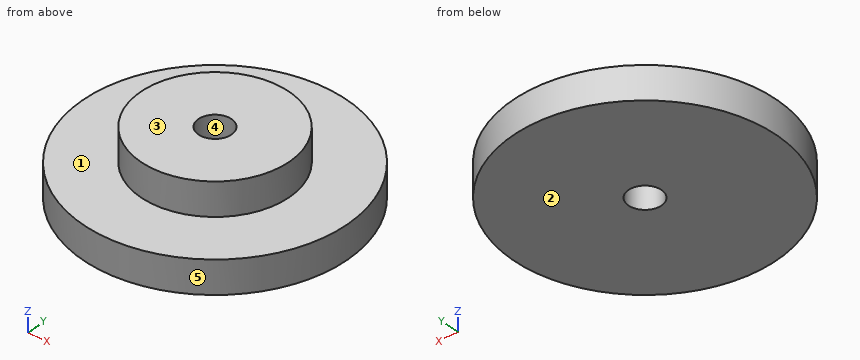
from build123d import *

# Parameters (mm, degrees)
F0_R     = 12.7
F0_R_2   = 7.14375
F1_DEPTH = 3.175
F0_R_3   = 1.5875
F2_DEPTH = 6.35
F3_DEPTH = 6.35


with BuildPart() as f1:
    # F0 (on Top) → F1 (new body)
    with BuildSketch(Plane.XY):
        Circle(F0_R)
        Circle(F0_R_2, mode=Mode.SUBTRACT)
    extrude(amount=F1_DEPTH)

    # F0 (on Top) → F2 (join)
    with BuildSketch(Plane.XY):
        Circle(F0_R_2)
        Circle(F0_R_3, mode=Mode.SUBTRACT)
    extrude(amount=F2_DEPTH)

    # F0 (on Top) → F3 (cut)
    with BuildSketch(Plane.XY):
        Circle(F0_R_3)
    extrude(amount=-F3_DEPTH, mode=Mode.SUBTRACT)


solid = f1.part
Build history of the part. All positions in model axes, mm. Face numbers are marked on the shaded views. A direction names the side the tool comes from. Coordinates: 2 decimals unless noted, no trailing zeros. Write each loop counter-clockwise with the first axis right and the second up, starting at its lowest first coordinate (ties: lowest second). Pieces come first, ordered by that corner, then holes.
(1) Cut at C-C on z = 1.75. List the corners of the cut face in (x, y) (1 decimal).
(2) 3-axis set-ups, long thin cutter, end or side, ignore diameter. For the marked faces 1 and 2: which of +Z, -Z, +X, -X, +Y, -Y reach the whole face in a straight line?
(3) Mould opens along X. For the marked faces 3, 4 and 5 say: pulls with the +X half, pulls with the -X half, needs draft (parallel to the pull), parting line crosses it, or undercut.
(4) Pin check, flat tips, straight feed: pin 1 Ø3 at (x, z) = (-7, 0.5) entering from -Y; pin 2 Ø1 at (x, y) = (0.5, 9) entering from +Z (3 decimals); pin 3 Ø1 at (y, z) = (9.5, 2.5) entering from +X. Stop position of each tip, or through.
(5) Drill centre lines: line 1 (Y direction, x = 0, z = 2.75); line 2 (Z direction, x = -6.75, y = -8.5) (3 decimals); line 3 (X direction, y = -10.5, z = 3). Where is each one in solid material? Low to high.
(6) Cut at D-D on x = 5.5. List the corners of the cut face in (y, z) (3 decimals).
Working result:
1. outline: circle Ø25.4 at (0, 0); hole circle Ø3.2 at (0, 0)
2. face 1: +Z
2. face 2: -Z, +X, -X, +Y, -Y
3. face 3: needs draft
3. face 4: undercut
3. face 5: parting line crosses it
4. pin 1: stops at y = -11.45
4. pin 2: stops at z = 3.175
4. pin 3: stops at x = 8.96
5. line 1: y = -12.7 to -1.59, 1.59 to 12.7
5. line 2: z = 0 to 3.175
5. line 3: x = -7.14 to 7.14
6. outline: (-11.447, 0) - (11.447, 0) - (11.447, 3.175) - (4.559, 3.175) - (4.559, 6.35) - (-4.559, 6.35) - (-4.559, 3.175) - (-11.447, 3.175) - close
